from build123d import *

# Parameters (mm, degrees)
CROQUIS1_W              = 75
CROQUIS1_H              = 160
CROQUIS1_R              = 12.5
CROQUIS1_R_2            = 3
SALIENTE_EXTRUIR1_DEPTH = 3
REDONDEO1_R             = 6


with BuildPart() as part:
    # Croquis1 → Saliente-Extruir1 (new body)
    with BuildSketch(Plane.XY):
        Rectangle(CROQUIS1_W, CROQUIS1_H)
        with Locations((0, 55)):
            Circle(CROQUIS1_R, mode=Mode.SUBTRACT)
        with Locations((0, -55)):
            Circle(CROQUIS1_R, mode=Mode.SUBTRACT)
        with Locations((-29.5, 72)):
            Circle(CROQUIS1_R_2, mode=Mode.SUBTRACT)
        with Locations((29.5, 72)):
            Circle(CROQUIS1_R_2, mode=Mode.SUBTRACT)
        with Locations((-29.5, -72)):
            Circle(CROQUIS1_R_2, mode=Mode.SUBTRACT)
        with Locations((29.5, -72)):
            Circle(CROQUIS1_R_2, mode=Mode.SUBTRACT)
    extrude(amount=SALIENTE_EXTRUIR1_DEPTH)

    # Redondeo1
    redondeo1_edges = [part.edges().sort_by_distance(p)[0] for p in [
        (-37.5, 80, 1.5),
        (37.5, 80, 1.5),
        (37.5, -80, 1.5),
        (-37.5, -80, 1.5),
    ]]
    fillet(redondeo1_edges, radius=REDONDEO1_R)


solid = part.part
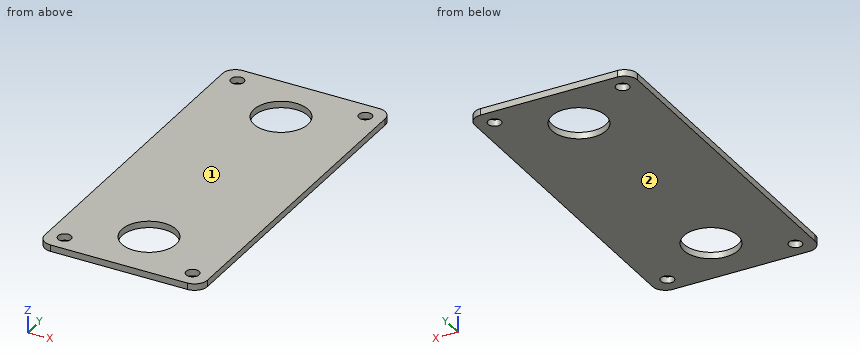
Could you check a few things on this model? Use its own coordinates, in mm. Face numbers are marked on the shaded views. Give positions to 0.01 mm unless a question says otherwise; leave off trailing zeros. Write each loop counter-clockwise with the first axis right and the second up, starting at its lowest first coordinate (ties: lowest second). Pieces come first, ordered by that corner, then holes. Notation, with made-up numbers: (63, 80) -> (88, 80) arc R34 cw to (88, 113) -> close; hole circle Ø5 at (81.25, 87.25). An arc over 180 degrees is marked (long way). Write each question's results on one line, items separated by ' | '. Start each with the question number.
Q1. We'd pull the mould along Z, two halves only. Please class the marked faces 1 and 2: +Z half, -Z half, draft (parallel to the pull), parting line (faces both ways), or undercut.
Q2. Suppose I cut it at D-D, the plane y = 72. List the corners of the cut face in (x, z) for me, and give its area (3 significant figures).
Q3. Suppose I cut it at C-C, the plane z = 1.95. List the corners of the cut face in (x, y) for me.
Q4. I'm going to push flat-ended pins straight in: pin 1 Ø22.5 at (x, y) = (0, -55) entering from +Z; pin 2 Ø8 at (x, y) = (-29.5, -72) entering from +Z. Where does each tip first touch, or does it pass through?
Q5. Suppose I cut it at B-B, the plane x = -29.5. List the corners of the cut face in (y, z) for me.
Q6. Suppose I cut it at A-A, the plane y = -55. List the corners of the cut face in (x, z) for me.
Q7. I need wall thicknesses on probe 1 along Y at (x, z) = (-29.5, 1.2); probe 2 along X at (y, z) = (57, 0.45); probe 3 along X at (y, z) = (-54, 0.45). Which ranges of each line are inside material? Lowest first, please.
Outcome:
1) face 1: +Z half | face 2: -Z half
2) outline: (-37.5, 0) -> (-32.5, 0) -> (-32.5, 3) -> (-37.5, 3) -> close; (-26.5, 0) -> (26.5, 0) -> (26.5, 3) -> (-26.5, 3) -> close; (32.5, 0) -> (37.5, 0) -> (37.5, 3) -> (32.5, 3) -> close | area: 189 mm2
3) outline: (-37.5, -74) arc R6 ccw to (-31.5, -80) -> (31.5, -80) arc R6 ccw to (37.5, -74) -> (37.5, 74) arc R6 ccw to (31.5, 80) -> (-31.5, 80) arc R6 ccw to (-37.5, 74) -> close; hole circle Ø6 at (-29.5, -72); hole circle Ø6 at (-29.5, 72); hole circle Ø25 at (0, -55); hole circle Ø25 at (0, 55); hole circle Ø6 at (29.5, -72); hole circle Ø6 at (29.5, 72)
4) pin 1: through | pin 2: z = 3
5) outline: (-80, 0) -> (-75, 0) -> (-75, 3) -> (-80, 3) -> close; (-69, 0) -> (69, 0) -> (69, 3) -> (-69, 3) -> close; (75, 0) -> (80, 0) -> (80, 3) -> (75, 3) -> close
6) outline: (-37.5, 0) -> (-12.5, 0) -> (-12.5, 3) -> (-37.5, 3) -> close; (12.5, 0) -> (37.5, 0) -> (37.5, 3) -> (12.5, 3) -> close
7) probe 1: -80 to -75, -69 to 69, 75 to 80 | probe 2: -37.5 to -12.34, 12.34 to 37.5 | probe 3: -37.5 to -12.46, 12.46 to 37.5
